Input: part model. Units: mm. Frame: model coordinates. A direction names the side the tool comes from. Coordinates: 2 decimals unless noted, no trailing zeros. Loops run counter-clockwise (first coordinate to the right, second up) from the corner with the lowest first, then second, coordinate; pieces in that order, holes last. Notation, with made-up numbers: (39, 35.5) - (59, 35.5) arc R11 cw to (59, 56.5) - close; hole circle Ø6 at (87.5, 25). An arc over 180 degrees is marked (long way). Use one line per item in the form item = value.
from build123d import *

# Parameters (mm, degrees)
SKETCH_1_W      = 15
SKETCH_1_H      = 15
EXTRUDE_1_DEPTH = 9
SKETCH_5_R      = 7.5
EXTRUDE_2_DEPTH = 7
SKETCH_6_R      = 8
EXTRUDE_3_DEPTH = 3
FILLET_1_R      = 3


with BuildPart() as part:
    # 草图1 → 凸台-拉伸1 (new body)
    with BuildSketch(Plane.XY):
        Rectangle(SKETCH_1_W, SKETCH_1_H)
    extrude(amount=EXTRUDE_1_DEPTH)

    # 草图5 → 凸台-拉伸2 (add)
    with BuildSketch(Plane.XY.offset(9)):
        Circle(SKETCH_5_R)
    extrude(amount=EXTRUDE_2_DEPTH)

    # 草图6 → 凸台-拉伸3 (add)
    with BuildSketch(Plane.XY.offset(16)):
        Circle(SKETCH_6_R)
    extrude(amount=EXTRUDE_3_DEPTH)

    # 圆角1
    fillet_1_edges = [part.edges().sort_by_distance(p)[0] for p in [
        (-8, 0, 19),
    ]]
    fillet(fillet_1_edges, radius=FILLET_1_R - 0.0001)  # a hair under: the kernel refuses the full size


solid = part.part
Q1. Cut plane B-B, the plane z = 6.25. Return loops of the section in (x, y).
Check values:
outline = (-7.5, -7.5) - (7.5, -7.5) - (7.5, 7.5) - (-7.5, 7.5) - close
Q2. Cut plane A-A, the plane z = 11. Return loops of the section in (x, y).
Check values:
outline = circle Ø15 at (0, 0)
Q3. Ray query, line 1 along Y through (x, z) = (-4, 4.25); line 2 along Z through (x, y) = (-4, -3.25). Return the intervals inside material, ascending. Write a range as [from, to].
Check values:
line_1 = [-7.5, 7.5]
line_2 = [0, 19]
Q4. Pull-direction query (Z, two-part tool) for faces 1 (the flat face through (6, -6, 9)), 2 (the flat face through (0, 0, 19)), 3 (the flat face through (7.5, 0, 4)); classes: pulls with the +Z half, pulls with the -Z half, needs draft (parallel to the pull), parting line crosses it, or undercut.
Check values:
face_1 = undercut
face_2 = pulls with the +Z half
face_3 = needs draft
Q5. Set-up query: faces 4 (the flat face through (-6, 6, 9)), 5 (the flat face through (0, 7.5, 4)), 6 (the flat face through (5, -6, 16)). Return all of +Z, -Z, +X, -X, +Y, -Y with unobstructed straight access to the full face (end or side cutting, diameter ignored); none if empty.
Check values:
face_4 = -X, +Y
face_5 = -Z, +X, -X, +Y
face_6 = none
Q6. First-contact query: P1, Ø6, axis at x = -1.5, z = 10, coming from the -Y side; P2, Ø1.5, axis at x = -2.5, y = -4.5, coming from the +Z side; P3, Ø7, axis at y = -0.5, z = 3.5, coming from the -X side. Flat tips, straight axial feed; report the tip coordinate or a pass-through.
Check values:
P1 = -7.5
P2 = 19
P3 = -7.5
